Verification items for the finished model (mm, model axes). A direction names the side the tool comes from. Coordinates: 2 decimals unless noted, no trailing zeros. Write each loop counter-clockwise with the first axis right and the second up, starting at its lowest first coordinate (ties: lowest second). Pieces come first, ordered by that corner, then holes. Notation, with made-up numbers: M -14.75,1 L -9.75,1 A25 cw -9.75,18 Z; hole C 18,58 d7. An arc over 180 degrees is marked long. One line per item, written item: value.
```python
from build123d import *

# Parameters (mm, degrees)
CROQUIS1_W                   = 300
CROQUIS1_H                   = 250
SALIENTE_EXTRUIR1_DEPTH      = 500
CROQUIS3_W                   = 500
CROQUIS3_H                   = 25
SALIENTE_EXTRUIR2_DEPTH      = 25
SALIENTE_EXTRUIR2_DEPTH_BACK = 325
VACIADO1_T                   = -5


with BuildPart() as part:
    # Croquis1 → Saliente-Extruir1 (new body)
    with BuildSketch(Plane.XY):
        Rectangle(CROQUIS1_W, CROQUIS1_H)
    extrude(amount=SALIENTE_EXTRUIR1_DEPTH)

    # Croquis3 → Saliente-Extruir2 (add, two sides)
    with BuildSketch(Plane(origin=(150, 0, 0), x_dir=(0, 0, -1), z_dir=(1, 0, 0))) as saliente_extruir2_sk:
        with Locations((-250, -17.5)):
            Rectangle(CROQUIS3_W, CROQUIS3_H)
    extrude(amount=SALIENTE_EXTRUIR2_DEPTH)
    extrude(saliente_extruir2_sk.sketch, amount=-SALIENTE_EXTRUIR2_DEPTH_BACK)

    # Vaciado1
    vaciado1_openings = [part.faces().sort_by_distance(p)[0] for p in [
        (0, 125, 250),
    ]]
    offset(amount=VACIADO1_T, openings=vaciado1_openings, kind=Kind.INTERSECTION)


solid = part.part
```
Item 1: Cross-section at D-D, the plane y = -19.5. Enter the section's corners in (x, z).
The answers:
outline: M -175,0 L 175,0 L 175,500 L -175,500 Z; hole M -170,5 L 170,5 L 170,495 L -170,495 Z
Item 2: Scan lines: line 1 (Z direction, x = 9, y = 63); line 2 (X direction, y = 15, z = 90); line 3 (X direction, y = -14, z = 67). Record each from-to range of solid material in increasing order.
The answers:
line 1: z = 0 to 5, 495 to 500
line 2: x = -150 to -145, 145 to 150
line 3: x = -175 to -170, 170 to 175
Item 3: Draft check along Z on faces 6 (the face through (-162, -30, 253)), 7 (the face through (2, -2, 500)), 8 (the face through (157, -10, 253)). Enter one of: released by +Z, released by -Z, zero draft, split by the parting line, or undercut.
The answers:
face 6: zero draft
face 7: released by +Z
face 8: undercut
Item 4: Go/stop test with flat-tipped pins: P1, Ø7.5, axis at x = 154, z = 142, coming from the +Y side; P2, Ø4, axis at x = 76, z = 431.5, coming from the +Y side; P3, Ø1.5, axis at y = -62.5, z = 273, coming from the +X side. Record where each tip stops, or that it passes through.
The answers:
P1: stops at y = -5
P2: stops at y = -120
P3: stops at x = 150
Item 5: Cross-section at C-C, the plane x = 13.5. Enter the section's corners in (y, z), and give its area (3 significant figures).
The answers:
outline: M -125,0 L 125,0 L 125,5 L -120,5 L -120,495 L 125,495 L 125,500 L -125,500 Z
area: 4,950 mm²
Item 6: Access from +Z, -Z, +X, -X, +Y, -Y to the whole of each face (thin tool, end or side, straight path). Record for faces 1 (the face through (-162, -5, 253)), 2 (the face through (150, -78, 246)), 3 (the face through (175, -17, 253)), 4 (the face through (-145, 57, 247)), 5 (the face through (-157, -10, 253)).
The answers:
face 1: +Z, -Z, -X, +Y
face 2: +Z, -Z, +X, -Y
face 3: +Z, -Z, +X, +Y, -Y
face 4: +Y
face 5: none
Item 7: Cross-section at A-A, the plane y = 62. Enter the section's corners in (x, z), and give its area (3 significant figures).
The answers:
outline: M -150,0 L 150,0 L 150,500 L -150,500 Z; hole M -145,5 L 145,5 L 145,495 L -145,495 Z
area: 7,900 mm²
Item 8: Cross-section at B-B, the plane z = 339. Enter the section's corners in (x, y).
The answers:
outline: M -175,-30 L -150,-30 L -150,-125 L 150,-125 L 150,-30 L 175,-30 L 175,-5 L 150,-5 L 150,125 L 145,125 L 145,-10 L 170,-10 L 170,-25 L 145,-25 L 145,-120 L -145,-120 L -145,-25 L -170,-25 L -170,-10 L -145,-10 L -145,125 L -150,125 L -150,-5 L -175,-5 Z
